Here's the drawing with two shaded views (mm, measured from the low corner). I have some questions. A direction names the side the tool comes from. Give positions to 0.01 mm unless a question says otherwise; leave off trailing zeros. Write each loop counter-clockwise with the first axis right and the second up, starting at its lowest first coordinate (ties: lowest second). Pieces come first, ordered by that corner, then holes. Notation, with made-up numbers: (-36, 31) - (-15, 31) arc R31 cw to (-15, 68) - close; hole circle Ø10 at (22, 14.5). An arc over 180 degrees is marked (long way). Write item = value, one per line.
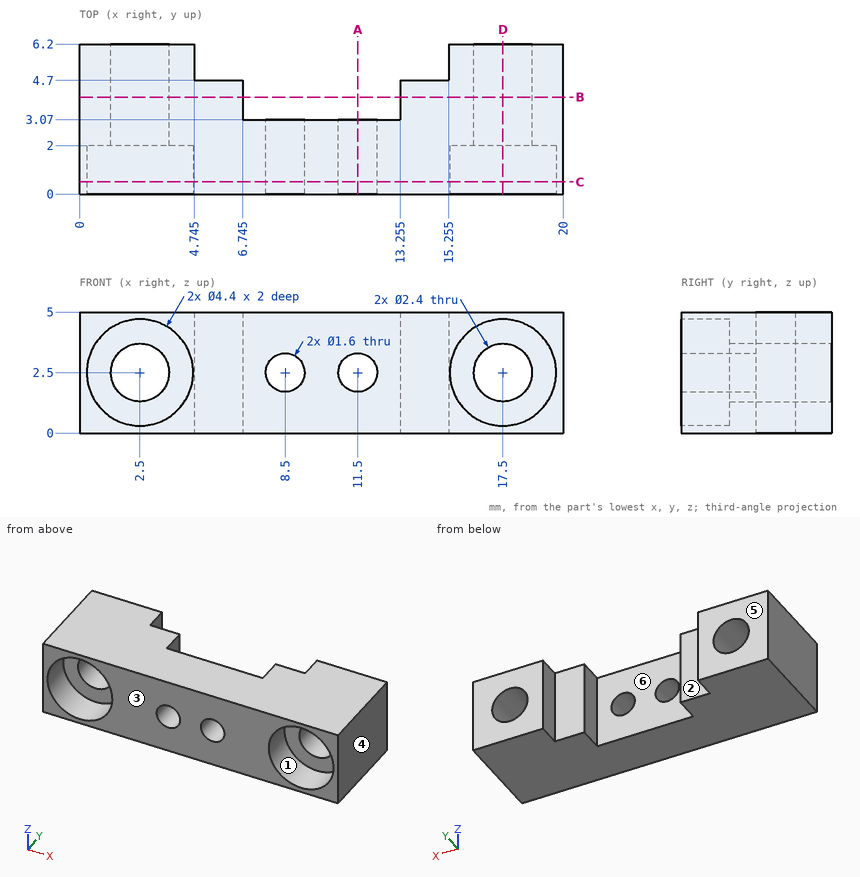
1. If we section it at C-C, the plane y = 0.5: Please give me the cut outline in (x, z), and give its area (3 significant figures).
Filled sheet:
outline = (0, 0) - (20, 0) - (20, 5) - (0, 5) - close; hole circle Ø4.4 at (2.5, 2.5); hole circle Ø1.6 at (8.5, 2.5); hole circle Ø1.6 at (11.5, 2.5); hole circle Ø4.4 at (17.5, 2.5)
area = 65.6 mm2
2. If we section it at B-B, the plane y = 4: Please give me the cut outline in (x, z) (3 decimals), and give its area (3 significant figures).
Filled sheet:
outline = (0, 0) - (6.745, 0) - (6.745, 5) - (0, 5) - close; (13.255, 0) - (20, 0) - (20, 5) - (13.255, 5) - close; hole circle Ø2.4 at (2.5, 2.5); hole circle Ø2.4 at (17.5, 2.5)
area = 58.4 mm2
3. For pin 1 (0.6 mm diameter, centred on x = 5.5, z = 2, fed in from +Y); pin 2 (1 mm diameter, centred on x = 7, z = 4.5, fed in from -Y); pin 3 (1.8 mm diameter, centred on x = 11.5, z = 2.5, fed in from +Y), each with a flat end and sliding along its axis, tell me the tip position at first contact or that it passes through.
Filled sheet:
pin_1 = 4.7
pin_2 = 0
pin_3 = 3.07
4. Thinking about a two-plate mould opening in X: for the marked faces 4, 5 and 6, which applies, pulls with the +X half, pulls with the -X half, needs draft (parallel to the pull), parting line crosses it, or undercut?
Filled sheet:
face_4 = pulls with the +X half
face_5 = needs draft
face_6 = undercut
5. I need wall thicknesses on line 1 (X direction, y = 1.25, z = 2.5); line 2 (X direction, y = 2.4, z = 2.5); line 3 (X direction, y = 5.5, z = 4.3) (3 decimals). Which ranges of each line are inside material? Lowest first, please.
Filled sheet:
line_1 = 0 to 0.3, 4.7 to 7.7, 9.3 to 10.7, 12.3 to 15.3, 19.7 to 20
line_2 = 0 to 1.3, 3.7 to 7.7, 9.3 to 10.7, 12.3 to 16.3, 18.7 to 20
line_3 = 0 to 4.745, 15.255 to 20
6. If we section it at D-D, the plane x = 17.5: Please give me the cut outline in (y, z), and give its area (3 significant figures).
Filled sheet:
outline = (0, 0) - (6.2, 0) - (6.2, 1.3) - (2, 1.3) - (2, 0.3) - (0, 0.3) - close; (0, 4.7) - (2, 4.7) - (2, 3.7) - (6.2, 3.7) - (6.2, 5) - (0, 5) - close
area = 12.1 mm2
7. Which directions (+Z, -Z, +X, -X, +Y, -Y) give clear straight access to the entire face, cutting with the end or side of a thin tool? Please do the marked faces 1, 2 and 3.
Filled sheet:
face_1 = -Y
face_2 = +Z, -Z, +Y
face_3 = +Z, -Z, +X, -X, -Y
8. If we section it at A-A, the plane x = 11.5: Please give me the cut outline in (y, z), and give its area (3 significant figures).
Filled sheet:
outline = (0, 0) - (3.07, 0) - (3.07, 1.7) - (0, 1.7) - close; (0, 3.3) - (3.07, 3.3) - (3.07, 5) - (0, 5) - close
area = 10.4 mm2
